Design review of the part built by this model. Coordinates are the model's own, in mm. A direction names the side the tool comes from. Coordinates: 2 decimals unless noted, no trailing zeros. Order: outer loops, then holes, each group sorted by start corner. A loop starts at its lowest first (then second) coordinate and runs counter-clockwise, first axis right, second up. Notation, with made-up numbers: (80, 1.25) -> (86, 1.25) arc R22 ccw to (86, 20.25) -> close; hole circle Ø4 at (-29.5, 15.5). An arc over 180 degrees is marked (long way). Write item = value, one per line.
```python
from build123d import *

# Parameters (mm, degrees)
F1_DEPTH = 63.5
F2_DEPTH = 25.4
F3_DEPTH = 7.9375


with BuildPart() as f1:
    # F0 (on Front) → F1 (new body, symmetric)
    with BuildSketch(Plane.XZ):
        Polygon((-41.275, -9.525), (41.275, -9.525), (41.275, 9.525), (22.225, 9.525), (-41.275, 9.525), align=None)
    extrude(amount=F1_DEPTH, both=True)

    # F0 (on Front) → F2 (join, symmetric)
    with BuildSketch(Plane.XZ):
        with BuildLine():
            Line((22.225, 9.525), (41.275, 9.525))
            Line((41.275, 9.525), (41.275, 27.0002))
            ThreePointArc((41.275, 27.0002), (45.92468, 38.22552), (57.15, 42.8752))
            Line((57.15, 42.8752), (60.325, 42.8752))
            Line((60.325, 42.8752), (60.325, 61.9252))
            Line((60.325, 61.9252), (57.15, 61.9252))
            ThreePointArc((57.15, 61.9252), (32.454296, 51.695904), (22.225, 27.0002))
            Line((22.225, 27.0002), (22.225, 9.525))
        make_face()
    extrude(amount=F2_DEPTH, both=True)

    # F0 (on Front) → F3 (join, symmetric)
    with BuildSketch(Plane.XZ):
        with BuildLine():
            add(Edge.make_bspline(
                [(-41.275, 9.525), (-26.669292, 46.137553), (18.325027, 62.395359), (60.325, 66.675)],
                knots=[0, 0, 0, 0, 116.570504, 116.570504, 116.570504, 116.570504], degree=3))
            Line((-41.275, 9.525), (22.225, 9.525))
            Line((22.225, 9.525), (22.225, 27.0002))
            ThreePointArc((22.225, 27.0002), (32.454296, 51.695904), (57.15, 61.9252))
            Line((57.15, 61.9252), (60.325, 61.9252))
            Line((60.325, 61.9252), (60.325, 66.675))
        make_face()
    extrude(amount=F3_DEPTH, both=True)


solid = f1.part
```
(1) We need section B-B (y = 47). Write out the cut boundary in (x, z) (3 decimals).
Report:
outline = (-41.275, -9.525) -> (41.275, -9.525) -> (41.275, 9.525) -> (-41.275, 9.525) -> close
(2) For faces 1 (the cylindrical face through (32.73, -16.79, 51.97)), 2 (the flat face through (59, 17, 61.925)), 3 (the flat face through (41.275, -1, 4)), 4 (the flat face through (37, -25.4, 36)), 5 (the flat face through (-1, 7.938, 32)), list the 3-axis set-ups (+Z, -Z, +X, -X, +Y, -Y) from which the entire face can be reached by the end or side of a thin tool; tool diameter is ignored.
Report:
face_1 = +Z, -X, -Y
face_2 = +Z, +X, -X, +Y
face_3 = -Z, +X, +Y, -Y
face_4 = +Z, +X, -X, -Y
face_5 = +Z, -X, +Y
(3) For L1, parallel to Z at x = 14, y = 21 (3 decimals); L2, parallel to X at y = -13, z = 14 (3 decimals); L3, parallel to Y at x = 27.5, z = 29, list the stretches that pass through material, from the lowest coordinate up.
Report:
L1 = -9.525 to 9.525
L2 = 22.225 to 41.275
L3 = -25.4 to 25.4
(4) We need section A-A (y = -15). Write out the cut boundary in (x, z) (3 decimals), and give its area (3 significant figures).
Report:
outline = (-41.275, -9.525) -> (41.275, -9.525) -> (41.275, 27) arc R15.875 cw to (57.15, 42.875) -> (60.325, 42.875) -> (60.325, 61.925) -> (57.15, 61.925) arc R34.925 ccw to (22.225, 27) -> (22.225, 9.525) -> (-41.275, 9.525) -> close
area = 2,730 mm²
(5) Insertion check: pin 1 (2.5 mm diameter, centred on x = 59, y = -19, fed in from +Z); pin 2 (1 mm diameter, centred on x = -2, y = -31, fed in from +Z) (3 decimals); pin 3 (11.5 mm diameter, centred on x = 35.5, z = 47, fed in from -Y). Each pin has a flat end and moves straight along its axis. Give the tip position at first contact, or say it passes through.
Report:
pin_1 = 61.93
pin_2 = 9.525
pin_3 = -25.4
